```python
from build123d import *

# Parameters (mm, degrees)
BOX034_W        = 6
BOX034_H        = 1
BOX034_DEPTH    = 2
BOX033_W        = 1
BOX033_H        = 3.5
BOX033_DEPTH    = 2
BOX032_W        = 1
BOX032_H        = 3.5
BOX032_DEPTH    = 2
BOX031_W        = 6
BOX031_H        = 3.5
BOX031_DEPTH    = 2
BOX035_W        = 6
BOX035_H        = 1
BOX035_DEPTH    = 2
CHAMFER003_SIZE = 0.9
BOX024_W        = 6
BOX024_H        = 1
BOX024_DEPTH    = 2
BOX023_W        = 1
BOX023_H        = 3.5
BOX023_DEPTH    = 2
BOX022_W        = 1
BOX022_H        = 3.5
BOX022_DEPTH    = 2
BOX017_W        = 6
BOX017_H        = 3.5
BOX017_DEPTH    = 2
BOX025_W        = 6
BOX025_H        = 1
BOX025_DEPTH    = 2
CHAMFER001_SIZE = 0.9
BOX014_W        = 6
BOX014_H        = 3.5
BOX014_DEPTH    = 3
BOX015_W        = 6
BOX015_H        = 3.5
BOX015_DEPTH    = 3
BOX001_W        = 26
BOX001_H        = 26
BOX001_DEPTH    = 26
BOX_W           = 30
BOX_H           = 30
BOX_DEPTH       = 30
BOX029_W        = 6
BOX029_H        = 1
BOX029_DEPTH    = 2
BOX028_W        = 1
BOX028_H        = 3.5
BOX028_DEPTH    = 2
BOX027_W        = 1
BOX027_H        = 3.5
BOX027_DEPTH    = 2
BOX026_W        = 6
BOX026_H        = 3.5
BOX026_DEPTH    = 2
BOX030_W        = 6
BOX030_H        = 1
BOX030_DEPTH    = 2
CHAMFER002_SIZE = 0.9
BOX020_W        = 6
BOX020_H        = 1
BOX020_DEPTH    = 2
BOX019_W        = 1
BOX019_H        = 3.5
BOX019_DEPTH    = 2
BOX018_W        = 1
BOX018_H        = 3.5
BOX018_DEPTH    = 2
BOX016_W        = 6
BOX016_H        = 3.5
BOX016_DEPTH    = 2
BOX021_W        = 6
BOX021_H        = 1
BOX021_DEPTH    = 2
CHAMFER_SIZE    = 0.9


with BuildPart() as button2_box0010:
    # Box034 → Box034 (new body)
    with BuildSketch(Plane(origin=(12, 18, 28), x_dir=(1, 0, 0), z_dir=(0, 0, 1))):
        with Locations((3, 0.5)):
            Rectangle(BOX034_W, BOX034_H)
    extrude(amount=BOX034_DEPTH)


with BuildPart() as button2_box0009:
    # Box033 → Box033 (new body)
    with BuildSketch(Plane(origin=(18, 19, 28), x_dir=(1, 0, 0), z_dir=(0, 0, 1))):
        with Locations((0.5, 1.75)):
            Rectangle(BOX033_W, BOX033_H)
    extrude(amount=BOX033_DEPTH)


with BuildPart() as button2_box0008:
    # Box032 → Box032 (new body)
    with BuildSketch(Plane(origin=(11, 19, 28), x_dir=(1, 0, 0), z_dir=(0, 0, 1))):
        with Locations((0.5, 1.75)):
            Rectangle(BOX032_W, BOX032_H)
    extrude(amount=BOX032_DEPTH)


with BuildPart() as button2_box0007:
    # Box031 → Box031 (new body)
    with BuildSketch(Plane(origin=(12, 19, 28), x_dir=(1, 0, 0), z_dir=(0, 0, 1))):
        with Locations((3, 1.75)):
            Rectangle(BOX031_W, BOX031_H)
    extrude(amount=BOX031_DEPTH)


with BuildPart() as chamfer002bt2:
    # Box035 → Box035 (new body)
    with BuildSketch(Plane(origin=(12, 22.5, 28), x_dir=(1, 0, 0), z_dir=(0, 0, 1))):
        with Locations((3, 0.5)):
            Rectangle(BOX035_W, BOX035_H)
    extrude(amount=BOX035_DEPTH)

    # Fusion008: union Button2_box0010, Button2_box0009, Button2_box0008, Button2_box0007
    add(button2_box0010.part)
    add(button2_box0009.part)
    add(button2_box0008.part)
    add(button2_box0007.part)


with BuildPart() as chamfer002bt2_1:
    # Fusion008 placement: moved
    add(chamfer002bt2.part.moved(Location((0, 0, 1))))

    # Chamfer003
    chamfer003_edges = [chamfer002bt2_1.edges().sort_by_distance(p)[0] for p in [
        (11, 20.75, 31),
        (15, 18, 31),
        (15, 23.5, 31),
        (19, 20.75, 31),
    ]]
    chamfer(chamfer003_edges, length=CHAMFER003_SIZE)


with BuildPart() as chamfer002bt2_2:
    # Chamfer003 placement: moved
    add(chamfer002bt2_1.part.moved(Location((0, 0, -0.5))))


with BuildPart() as button2_box0005:
    # Box024 → Box024 (new body)
    with BuildSketch(Plane(origin=(12, 18, 28), x_dir=(1, 0, 0), z_dir=(0, 0, 1))):
        with Locations((3, 0.5)):
            Rectangle(BOX024_W, BOX024_H)
    extrude(amount=BOX024_DEPTH)


with BuildPart() as button2_box0004:
    # Box023 → Box023 (new body)
    with BuildSketch(Plane(origin=(18, 19, 28), x_dir=(1, 0, 0), z_dir=(0, 0, 1))):
        with Locations((0.5, 1.75)):
            Rectangle(BOX023_W, BOX023_H)
    extrude(amount=BOX023_DEPTH)


with BuildPart() as button2_box0003:
    # Box022 → Box022 (new body)
    with BuildSketch(Plane(origin=(11, 19, 28), x_dir=(1, 0, 0), z_dir=(0, 0, 1))):
        with Locations((0.5, 1.75)):
            Rectangle(BOX022_W, BOX022_H)
    extrude(amount=BOX022_DEPTH)


with BuildPart() as button2_box0002:
    # Box017 → Box017 (new body)
    with BuildSketch(Plane(origin=(12, 19, 28), x_dir=(1, 0, 0), z_dir=(0, 0, 1))):
        with Locations((3, 1.75)):
            Rectangle(BOX017_W, BOX017_H)
    extrude(amount=BOX017_DEPTH)


with BuildPart() as cut003:
    # Box025 → Box025 (new body)
    with BuildSketch(Plane(origin=(12, 22.5, 28), x_dir=(1, 0, 0), z_dir=(0, 0, 1))):
        with Locations((3, 0.5)):
            Rectangle(BOX025_W, BOX025_H)
    extrude(amount=BOX025_DEPTH)

    # Fusion003: union Button2_box0005, Button2_box0004, Button2_box0003, Button2_box0002
    add(button2_box0005.part)
    add(button2_box0004.part)
    add(button2_box0003.part)
    add(button2_box0002.part)


with BuildPart() as cut003_1:
    # Fusion003 placement: moved
    add(cut003.part.moved(Location((0, 0, 1))))

    # Chamfer001
    chamfer001_edges = [cut003_1.edges().sort_by_distance(p)[0] for p in [
        (11, 20.75, 31),
        (15, 18, 31),
        (15, 23.5, 31),
        (19, 20.75, 31),
    ]]
    chamfer(chamfer001_edges, length=CHAMFER001_SIZE)

    # Cut003: cut Chamfer002Bt2
    add(chamfer002bt2_2.part, mode=Mode.SUBTRACT)


with BuildPart() as button1_box0001:
    # Box014 → Box014 (new body)
    with BuildSketch(Plane(origin=(12, 7, 27), x_dir=(1, 0, 0), z_dir=(0, 0, 1))):
        with Locations((3, 1.75)):
            Rectangle(BOX014_W, BOX014_H)
    extrude(amount=BOX014_DEPTH)


with BuildPart() as fusion004_cut:
    # Box015 → Box015 (new body)
    with BuildSketch(Plane(origin=(12, 19, 27), x_dir=(1, 0, 0), z_dir=(0, 0, 1))):
        with Locations((3, 1.75)):
            Rectangle(BOX015_W, BOX015_H)
    extrude(amount=BOX015_DEPTH)

    # Fusion004: union Button1_box0001
    add(button1_box0001.part)


with BuildPart() as box_in:
    # Box001 → Box001 (new body)
    with BuildSketch(Plane(origin=(2, 2, 2), x_dir=(1, 0, 0), z_dir=(0, 0, 1))):
        with Locations((13, 13)):
            Rectangle(BOX001_W, BOX001_H)
    extrude(amount=BOX001_DEPTH)


with BuildPart() as cut001:
    # Box → Box (new body)
    with BuildSketch(Plane.XY):
        with Locations((15, 15)):
            Rectangle(BOX_W, BOX_H)
    extrude(amount=BOX_DEPTH)

    # Cut: cut Box_in
    add(box_in.part, mode=Mode.SUBTRACT)

    # Cut001: cut Fusion004_cut
    add(fusion004_cut.part, mode=Mode.SUBTRACT)


with BuildPart() as button1_box0010:
    # Box029 → Box029 (new body)
    with BuildSketch(Plane(origin=(12, 6, 28), x_dir=(1, 0, 0), z_dir=(0, 0, 1))):
        with Locations((3, 0.5)):
            Rectangle(BOX029_W, BOX029_H)
    extrude(amount=BOX029_DEPTH)


with BuildPart() as button1_box0009:
    # Box028 → Box028 (new body)
    with BuildSketch(Plane(origin=(18, 7, 28), x_dir=(1, 0, 0), z_dir=(0, 0, 1))):
        with Locations((0.5, 1.75)):
            Rectangle(BOX028_W, BOX028_H)
    extrude(amount=BOX028_DEPTH)


with BuildPart() as button1_box0008:
    # Box027 → Box027 (new body)
    with BuildSketch(Plane(origin=(11, 7, 28), x_dir=(1, 0, 0), z_dir=(0, 0, 1))):
        with Locations((0.5, 1.75)):
            Rectangle(BOX027_W, BOX027_H)
    extrude(amount=BOX027_DEPTH)


with BuildPart() as button1_box0007:
    # Box026 → Box026 (new body)
    with BuildSketch(Plane(origin=(12, 7, 28), x_dir=(1, 0, 0), z_dir=(0, 0, 1))):
        with Locations((3, 1.75)):
            Rectangle(BOX026_W, BOX026_H)
    extrude(amount=BOX026_DEPTH)


with BuildPart() as chamfer002bt1:
    # Box030 → Box030 (new body)
    with BuildSketch(Plane(origin=(12, 10.5, 28), x_dir=(1, 0, 0), z_dir=(0, 0, 1))):
        with Locations((3, 0.5)):
            Rectangle(BOX030_W, BOX030_H)
    extrude(amount=BOX030_DEPTH)

    # Fusion007: union Button1_box0010, Button1_box0009, Button1_box0008, Button1_box0007
    add(button1_box0010.part)
    add(button1_box0009.part)
    add(button1_box0008.part)
    add(button1_box0007.part)


with BuildPart() as chamfer002bt1_1:
    # Fusion007 placement: moved
    add(chamfer002bt1.part.moved(Location((0, 0, 1))))

    # Chamfer002
    chamfer002_edges = [chamfer002bt1_1.edges().sort_by_distance(p)[0] for p in [
        (11, 8.75, 31),
        (15, 6, 31),
        (15, 11.5, 31),
        (19, 8.75, 31),
    ]]
    chamfer(chamfer002_edges, length=CHAMFER002_SIZE)


with BuildPart() as chamfer002bt1_2:
    # Chamfer002 placement: moved
    add(chamfer002bt1_1.part.moved(Location((0, 0, -0.5))))


with BuildPart() as button1_box0005:
    # Box020 → Box020 (new body)
    with BuildSketch(Plane(origin=(12, 6, 28), x_dir=(1, 0, 0), z_dir=(0, 0, 1))):
        with Locations((3, 0.5)):
            Rectangle(BOX020_W, BOX020_H)
    extrude(amount=BOX020_DEPTH)


with BuildPart() as button1_box0004:
    # Box019 → Box019 (new body)
    with BuildSketch(Plane(origin=(18, 7, 28), x_dir=(1, 0, 0), z_dir=(0, 0, 1))):
        with Locations((0.5, 1.75)):
            Rectangle(BOX019_W, BOX019_H)
    extrude(amount=BOX019_DEPTH)


with BuildPart() as button1_box0003:
    # Box018 → Box018 (new body)
    with BuildSketch(Plane(origin=(11, 7, 28), x_dir=(1, 0, 0), z_dir=(0, 0, 1))):
        with Locations((0.5, 1.75)):
            Rectangle(BOX018_W, BOX018_H)
    extrude(amount=BOX018_DEPTH)


with BuildPart() as button1_box0002:
    # Box016 → Box016 (new body)
    with BuildSketch(Plane(origin=(12, 7, 28), x_dir=(1, 0, 0), z_dir=(0, 0, 1))):
        with Locations((3, 1.75)):
            Rectangle(BOX016_W, BOX016_H)
    extrude(amount=BOX016_DEPTH)


with BuildPart() as box:
    # Box021 → Box021 (new body)
    with BuildSketch(Plane(origin=(12, 10.5, 28), x_dir=(1, 0, 0), z_dir=(0, 0, 1))):
        with Locations((3, 0.5)):
            Rectangle(BOX021_W, BOX021_H)
    extrude(amount=BOX021_DEPTH)

    # Fusion002: union Button1_box0005, Button1_box0004, Button1_box0003, Button1_box0002
    add(button1_box0005.part)
    add(button1_box0004.part)
    add(button1_box0003.part)
    add(button1_box0002.part)


with BuildPart() as box_1:
    # Fusion002 placement: moved
    add(box.part.moved(Location((0, 0, 1))))

    # Chamfer
    chamfer_edges = [box_1.edges().sort_by_distance(p)[0] for p in [
        (11, 8.75, 31),
        (15, 6, 31),
        (15, 11.5, 31),
        (19, 8.75, 31),
    ]]
    chamfer(chamfer_edges, length=CHAMFER_SIZE)

    # Cut002: cut Chamfer002Bt1
    add(chamfer002bt1_2.part, mode=Mode.SUBTRACT)

    # Fusion009: union Cut003, Cut001
    add(cut003_1.part)
    add(cut001.part)


solid = box_1.part
```
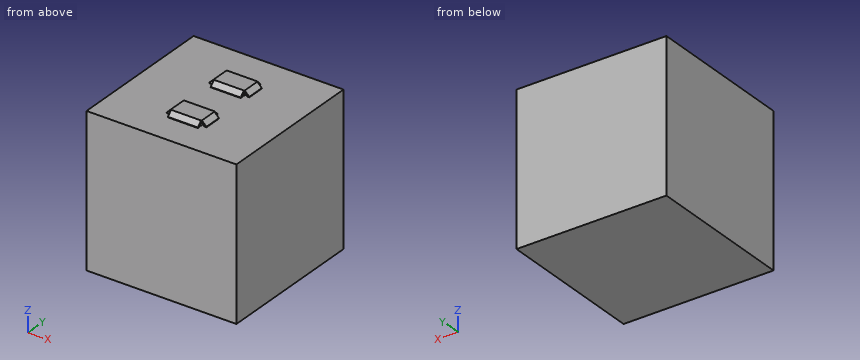
Geometry: final body of the model. Coordinates: model frame, mm. Give positions to 0.01 mm unless a question says otherwise; leave off trailing zeros. Loops run counter-clockwise (first coordinate to the right, second up) from the corner with the lowest first, then second, coordinate; pieces in that order, holes last. Notation, with made-up numbers: (58.5, -36) -> (114.5, -36) arc R13 cw to (114.5, -30) -> close; hole circle Ø3 at (-11.5, 81). An arc over 180 degrees is marked (long way). Return JSON: item names as keys, results as strings.
Item 1: Section B-B, the plane z = 16. Output: boundary loops of the cut face in (x, y), plus the area to 3 significant figures.
Filled in:
{"outline": "(0, 0) -> (30, 0) -> (30, 30) -> (0, 30) -> close; hole (2, 2) -> (28, 2) -> (28, 28) -> (2, 28) -> close", "area": "224 mm^2"}
Item 2: Pin query (flat end, axial travel): P1, Ø12, axis at x = 4.5, y = 10.5, coming from the +Z side; P2, Ø0.8, axis at y = 18.5, z = 30.5, coming from the -X side; P3, Ø0.8, axis at x = 18.5, z = 30.5, coming from the +Y side. Return the tip coordinate at first contact, or that it passes through.
Filled in:
{"P1": "z = 30", "P2": "x = 12", "P3": "y = 22.5"}
Item 3: Section A-A, the plane y = 8. Output: boundary loops of the cut face in (x, z).
Filled in:
{"outline": "(0, 0) -> (30, 0) -> (30, 30) -> (19, 30) -> (19, 30.1) -> (18.1, 31) -> (11.9, 31) -> (11, 30.1) -> (11, 30) -> (0, 30) -> close; hole (2, 2) -> (28, 2) -> (28, 28) -> (18, 28) -> (18, 30) -> (18.6, 30) -> (18.1, 30.5) -> (11.9, 30.5) -> (11.4, 30) -> (12, 30) -> (12, 28) -> (2, 28) -> close"}
Item 4: Line query: line 1 (X direction, y = 23, z = 23). Output: solid intervals per line, ascending.
Filled in:
{"line 1": "0 to 2, 28 to 30"}
